Drawing for the job (mm, zero at the part's lowest x, y, z). Give positions to 0.01 mm unless a question says otherwise; leave off trailing zeros. Write each loop counter-clockwise with the first axis right and the second up, starting at its lowest first coordinate (ties: lowest second). Pieces come first, ordered by that corner, then holes.
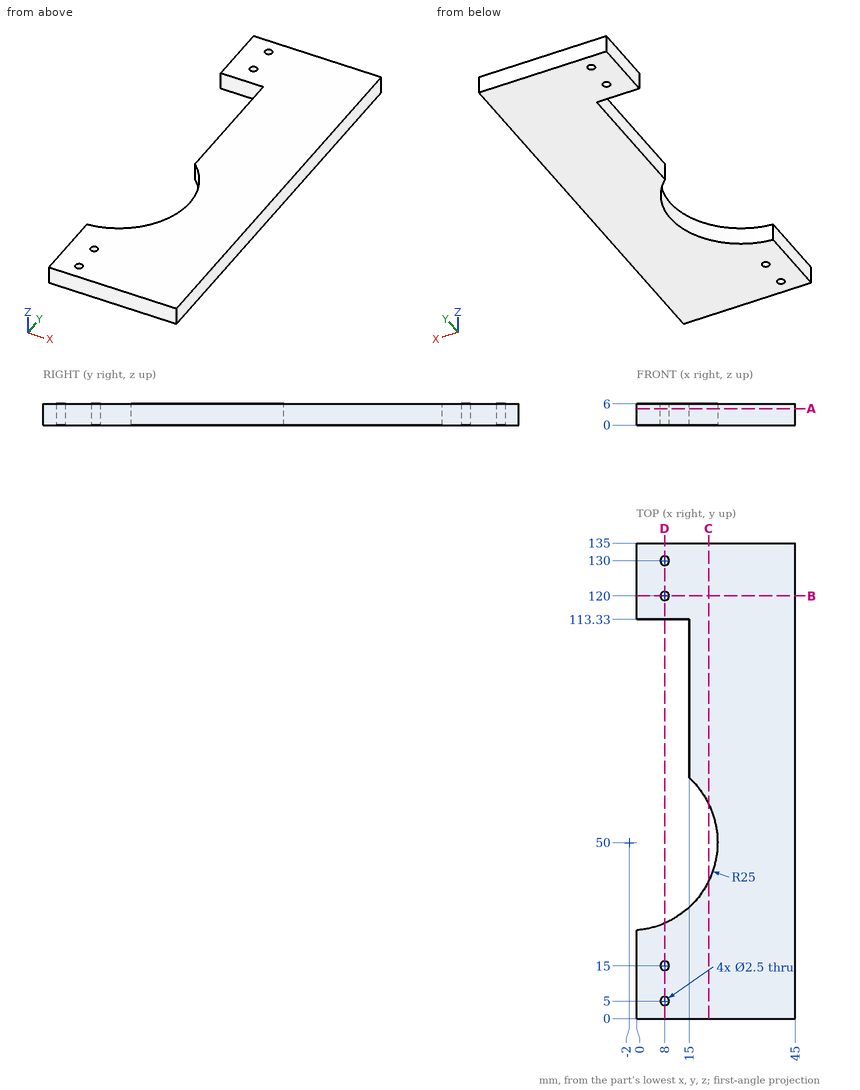
1. Probe probe 1 along X at (y, z) = (130, 3.85); probe 2 along Y at (x, z) = (8, 3.75); probe 3 along Y at (x, z) = (3.5, 4.1). List the from-to ranges inside material, lowest first.
Calculated:
probe 1: x = 0 to 6.75, 9.25 to 45
probe 2: y = 0 to 3.75, 6.25 to 13.75, 16.25 to 27.09, 113.33 to 118.75, 121.25 to 128.75, 131.25 to 135
probe 3: y = 0 to 25.61, 113.33 to 135
2. Slice it at D-D, the plane x = 8. Write the cut outline in (y, z).
Calculated:
outline: (0, 0) - (3.75, 0) - (3.75, 6) - (0, 6) - close; (6.25, 0) - (13.75, 0) - (13.75, 6) - (6.25, 6) - close; (16.25, 0) - (27.09, 0) - (27.09, 6) - (16.25, 6) - close; (113.33, 0) - (118.75, 0) - (118.75, 6) - (113.33, 6) - close; (121.25, 0) - (128.75, 0) - (128.75, 6) - (121.25, 6) - close; (131.25, 0) - (135, 0) - (135, 6) - (131.25, 6) - close
3. Slice it at A-A, the plane z = 4.7. Write the cut outline in (x, y).
Calculated:
outline: (0, 0) - (45, 0) - (45, 135) - (0, 135) - (0, 113.33) - (15, 113.33) - (15, 68.33) arc R25 cw to (0, 25.08) - close; hole circle Ø2.5 at (8, 5); hole circle Ø2.5 at (8, 15); hole circle Ø2.5 at (8, 120); hole circle Ø2.5 at (8, 130)
4. Pin check, flat tips, straight feed: P1, Ø1.5, axis at x = 8, y = 130, coming from the -Z side; P2, Ø1, axis at y = 76, z = 4.5, coming from the -X side. Stop position of each tip, or through.
Calculated:
P1: passes through
P2: stops at x = 15
5. Slice it at B-B, the plane y = 120. Write the cut outline in (x, z), and give its area (3 significant figures).
Calculated:
outline: (0, 0) - (6.75, 0) - (6.75, 6) - (0, 6) - close; (9.25, 0) - (45, 0) - (45, 6) - (9.25, 6) - close
area: 255 mm2
6. Slice it at C-C, the plane x = 20.5. Write the cut outline in (y, z).
Calculated:
outline: (0, 0) - (39.1, 0) - (39.1, 6) - (0, 6) - close; (60.9, 0) - (135, 0) - (135, 6) - (60.9, 6) - close
